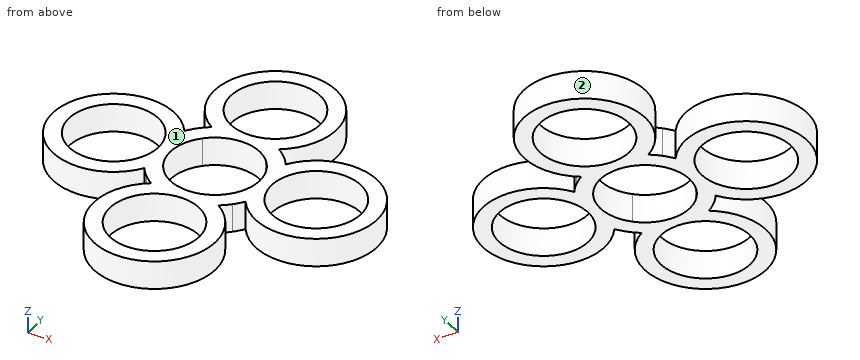
```python
from build123d import *

# Parameters (mm, degrees)
F0_R     = 11
F1_DEPTH = 7


with BuildPart() as f1:
    # F0 (on Top) → F1 (new body)
    with BuildSketch(Plane.XY):
        with BuildLine():
            ThreePointArc((10.606602, 10.606602), (9.496388, 11.611142), (8.291562, 12.5))
            ThreePointArc((8.291562, 12.5), (0, 40), (-8.291562, 12.5))
            ThreePointArc((-8.291562, 12.5), (-9.496388, 11.611142), (-10.606602, 10.606602))
            ThreePointArc((-10.606602, 10.606602), (-11.611142, 9.496388), (-12.5, 8.291562))
            ThreePointArc((-12.5, 8.291562), (-40, 0), (-12.5, -8.291562))
            ThreePointArc((-12.5, -8.291562), (-11.611142, -9.496388), (-10.606602, -10.606602))
            ThreePointArc((-10.606602, -10.606602), (-9.496388, -11.611142), (-8.291562, -12.5))
            ThreePointArc((-8.291562, -12.5), (0, -40), (8.291562, -12.5))
            ThreePointArc((8.291562, -12.5), (9.496388, -11.611142), (10.606602, -10.606602))
            ThreePointArc((10.606602, -10.606602), (11.611142, -9.496388), (12.5, -8.291562))
            ThreePointArc((12.5, -8.291562), (40, 0), (12.5, 8.291562))
            ThreePointArc((12.5, 8.291562), (11.611142, 9.496388), (10.606602, 10.606602))
        make_face()
        with Locations((0, -25)):
            Circle(F0_R, mode=Mode.SUBTRACT)
        with Locations((-25, 0)):
            Circle(F0_R, mode=Mode.SUBTRACT)
        with BuildLine():
            ThreePointArc((-7.778175, 7.778175), (0, 11), (7.778175, 7.778175))
            ThreePointArc((7.778175, 7.778175), (11, 0), (7.778175, -7.778175))
            ThreePointArc((7.778175, -7.778175), (0, -11), (-7.778175, -7.778175))
            ThreePointArc((-7.778175, -7.778175), (-11, 0), (-7.778175, 7.778175))
        make_face(mode=Mode.SUBTRACT)
        with Locations((25, 0)):
            Circle(F0_R, mode=Mode.SUBTRACT)
        with Locations((0, 25)):
            Circle(F0_R, mode=Mode.SUBTRACT)
    extrude(amount=F1_DEPTH)


solid = f1.part
```
Check sheet for the modelled part. Datum: model origin and axes. Units: mm. Face numbers are marked on the shaded views. Give positions to 0.01 mm unless a question says otherwise; leave off trailing zeros. Write each loop counter-clockwise with the first axis right and the second up, starting at its lowest first coordinate (ties: lowest second). Pieces come first, ordered by that corner, then holes. Notation, with made-up numbers: (59.5, 56.25) - (79.5, 56.25) arc R29 cw to (79.5, 78.25) - close; hole circle Ø1 at (74, 33). An arc over 180 degrees is marked (long way). Answer as a JSON object with one key per item and string values. Group by question number.
1) Sectioned sample at B-B (y = -25). Record the cut outline in (x, z), then the cut area to 3 significant figures.
2) Depth check by flat-ended pin: P1, Ø2, axis at x = -8, z = 6, coming from the -Y side; P2, Ø1.5, axis at x = 20, z = 5, coming from the +Y side; P3, Ø3, axis at y = -4, z = 5.5, coming from the +X side. Enter the tip coordinate at first touch or a pass-through.
3) Release check for a two-part mould opening along Y. For the marked faces 1 and 2 record: pulls with the +Y half, pulls with the -Y half, needs draft (parallel to the pull), parting line crosses it, or undercut.
4) Sectioned sample at D-D (z = 4.5). Record the cut outline in (x, y).
5) Thickness scan on probe 1 along Y at (x, z) = (25, 5); probe 2 along Y at (x, z) = (7.5, 3.25); probe 3 along X at (y, z) = (-3.5, 3). Record the ranges inside material, lowest first. Write a range as from..to.
6) Sectioned sample at A-A (x = 0). Record the cut outline in (y, z).
Geometry results:
{
 "1": {"outline": "(-15, 0) - (-11, 0) - (-11, 7) - (-15, 7) - close; (11, 0) - (15, 0) - (15, 7) - (11, 7) - close", "area": "56.0 mm^2"},
 "2": {"P1": "stops at y = -38.27", "P2": "stops at y = 14.39", "P3": "stops at x = 39.79"},
 "3": {"face 1": "needs draft", "face 2": "undercut"},
 "4": {"outline": "(-12.5, -8.29) arc R15 ccw to (-10.61, -10.61) arc R15 ccw to (-8.29, -12.5) arc R15 ccw (long way) to (8.29, -12.5) arc R15 ccw to (10.61, -10.61) arc R15 ccw to (12.5, -8.29) arc R15 ccw (long way) to (12.5, 8.29) arc R15 ccw to (10.61, 10.61) arc R15 ccw to (8.29, 12.5) arc R15 ccw (long way) to (-8.29, 12.5) arc R15 ccw to (-10.61, 10.61) arc R15 ccw to (-12.5, 8.29) arc R15 ccw (long way) to start; hole circle Ø22 at (-25, 0); hole circle Ø22 at (0, -25); hole circle Ø22 at (0, 25); hole (-7.78, -7.78) arc R11 ccw to (7.78, -7.78) arc R11 ccw to (7.78, 7.78) arc R11 ccw to (-7.78, 7.78) arc R11 ccw to start; hole circle Ø22 at (25, 0)"},
 "5": {"probe 1": "y = -15..-11, 11..15", "probe 2": "y = -37.99..-33.05, -16.95..-8.05, 8.05..16.95, 33.05..37.99", "probe 3": "x = -39.59..-35.43, -14.57..-10.43, 10.43..14.57, 35.43..39.59"},
 "6": {"outline": "(-40, 0) - (-36, 0) - (-36, 7) - (-40, 7) - close; (-14, 0) - (-11, 0) - (-11, 7) - (-14, 7) - close; (11, 0) - (14, 0) - (14, 7) - (11, 7) - close; (36, 0) - (40, 0) - (40, 7) - (36, 7) - close"}
}
